Build history of the part. All positions in model axes, mm. Face numbers are marked on the shaded views. A direction names the side the tool comes from. Give positions to 0.01 mm unless a question says otherwise; leave off trailing zeros. Order: outer loops, then holes, each group sorted by start corner. A loop starts at its lowest first (then second) coordinate and runs counter-clockwise, first axis right, second up. Notation, with made-up numbers: (58, -33.5) - (109, -33.5) arc R18 ccw to (109, -16.5) - close; hole circle Ø3 at (16.5, 53). An arc over 180 degrees is marked (long way). Answer in a Markdown table with one row per item.
```python
from build123d import *

# Parameters (mm, degrees)
F0_R     = 25
F1_DEPTH = 1.9
F2_R     = 1.05
F3_DEPTH = 25.4
F5_DEPTH = 5


with BuildPart() as f1:
    # F0 (on Top) → F1 (new body)
    with BuildSketch(Plane.XY):
        Circle(F0_R)
    extrude(amount=F1_DEPTH)

    # F2 (on Top) → F3 (cut)
    with BuildSketch(Plane.XY):
        Circle(F2_R)
    extrude(amount=F3_DEPTH, mode=Mode.SUBTRACT)

    # F4 (on face) → F5 (join)
    with BuildSketch(Plane.XY.offset(1.9)):
        with BuildLine():
            ThreePointArc((-8.4449654791, 14.1750681853), (-7.8625386646, 14.5062223114), (-7.267148147, 14.8134586714))
            Line((-7.267148147, 14.8134586714), (-6.6282985683, 17.5245980034))
            Line((-6.6282985683, 17.5245980034), (-13.8357791201, 20.8223729709))
            ThreePointArc((-13.8357791201, 20.8223729709), (-14.3152843529, 20.4956735409), (-14.7870786227, 20.1579340659))
            Line((-14.7870786227, 20.1579340659), (-7.7896110966, 16.9562503322))
            Line((-7.7896110966, 16.9562503322), (-8.4449654791, 14.1750681853))
        make_face()
        with BuildLine():
            ThreePointArc((-1.4583194007, 16.4354283341), (-0.7898885826, 16.4810823682), (-0.1201554013, 16.4995624996))
            Line((-0.1201554013, 16.4995624996), (1.631747451, 18.6650281904))
            Line((1.631747451, 18.6650281904), (-3.4311172084, 24.7634293809))
            ThreePointArc((-3.4311172084, 24.7634293809), (-4.0048860655, 24.6771328886), (-4.5764976809, 24.5775439981))
            Line((-4.5764976809, 24.5775439981), (0.3388442045, 18.6568392545))
            Line((0.3388442045, 18.6568392545), (-1.4583194007, 16.4354283341))
        make_face()
        with BuildLine():
            ThreePointArc((5.8171647201, 15.4405503341), (6.4392086206, 15.1916619348), (7.0506355953, 14.917725621))
            Line((7.0506355953, 14.917725621), (9.5686058756, 16.1086206327))
            Line((9.5686058756, 16.1086206327), (7.6531195462, 23.7997848984))
            ThreePointArc((7.6531195462, 23.7997848984), (7.0987290239, 23.9709834226), (6.5405147537, 24.1292699176))
            Line((6.5405147537, 24.1292699176), (8.4001872552, 16.6622123514))
            Line((8.4001872552, 16.6622123514), (5.8171647201, 15.4405503341))
        make_face()
        with BuildLine():
            ThreePointArc((11.9404880253, 11.3874819745), (12.3929415847, 10.8933465417), (12.8249617418, 10.3812502291))
            Line((12.8249617418, 10.3812502291), (15.6102845553, 10.3617031995))
            Line((15.6102845553, 10.3617031995), (17.2215621154, 18.1223011316))
            ThreePointArc((17.2215621154, 18.1223011316), (16.7963537699, 18.5170867049), (16.3620980272, 18.9018980039))
            Line((16.3620980272, 18.9018980039), (14.7977701984, 11.3674299434))
            Line((14.7977701984, 11.3674299434), (11.9404880253, 11.3874819745))
        make_face()
        with BuildLine():
            ThreePointArc((15.6988512365, 5.0789831515), (15.8921004786, 4.4374702679), (16.0591469276, 3.7886409118))
            Line((16.0591469276, 3.7886409118), (18.5601549312, 2.5625233696))
            Line((18.5601549312, 2.5625233696), (23.379063099, 8.8554733703))
            ThreePointArc((23.379063099, 8.8554733703), (23.167254658, 9.3956538681), (22.9429671184, 9.9307733739))
            Line((22.9429671184, 9.9307733739), (18.2644732712, 3.8211886228))
            Line((18.2644732712, 3.8211886228), (15.6988512365, 5.0789831515))
        make_face()
        with BuildLine():
            Line((18.1136734135, -4.4818859684), (16.3478644266, -2.2354705742))
            ThreePointArc((16.3478644266, -2.2354705742), (16.2436339688, -2.8973014145), (16.1126211118, -3.5543552028))
            Line((16.1126211118, -3.5543552028), (17.8339589977, -5.7441956409))
            Line((17.8339589977, -5.7441956409), (24.9060539105, -2.1652894973))
            ThreePointArc((24.9060539105, -2.1652894973), (24.9495966334, -1.5867034474), (24.9797001948, -1.0072627157))
            Line((24.9797001948, -1.0072627157), (18.1136734135, -4.4818859684))
        make_face()
        with BuildLine():
            Line((14.3752383867, -11.8972680768), (13.7589825736, -9.1071619365))
            ThreePointArc((13.7589825736, -9.1071619365), (13.3779165365, -9.6582270186), (12.9747930765, -10.1933676782))
            Line((12.9747930765, -10.1933676782), (13.5755287655, -12.9132062568))
            Line((13.5755287655, -12.9132062568), (21.5000952923, -12.7571902244))
            ThreePointArc((21.5000952923, -12.7571902244), (21.7903650088, -12.2547946855), (22.0688972917, -11.7457980712))
            Line((22.0688972917, -11.7457980712), (14.3752383867, -11.8972680768))
        make_face()
        with BuildLine():
            Line((7.7896110966, -16.9562503322), (8.4449654791, -14.1750681853))
            ThreePointArc((8.4449654791, -14.1750681853), (7.8625386646, -14.5062223114), (7.267148147, -14.8134586714))
            Line((7.267148147, -14.8134586714), (6.6282985683, -17.5245980034))
            Line((6.6282985683, -17.5245980034), (13.8357791201, -20.8223729709))
            ThreePointArc((13.8357791201, -20.8223729709), (14.3152843529, -20.4956735409), (14.7870786227, -20.1579340659))
            Line((14.7870786227, -20.1579340659), (7.7896110966, -16.9562503322))
        make_face()
        with BuildLine():
            Line((-0.3388442045, -18.6568392545), (1.4583194007, -16.4354283341))
            ThreePointArc((1.4583194007, -16.4354283341), (0.7898885826, -16.4810823682), (0.1201554013, -16.4995624996))
            Line((0.1201554013, -16.4995624996), (-1.631747451, -18.6650281904))
            Line((-1.631747451, -18.6650281904), (3.4311172084, -24.7634293809))
            ThreePointArc((3.4311172084, -24.7634293809), (4.0048860655, -24.6771328886), (4.5764976809, -24.5775439981))
            Line((4.5764976809, -24.5775439981), (-0.3388442045, -18.6568392545))
        make_face()
        with BuildLine():
            Line((-8.4001872552, -16.6622123514), (-5.8171647201, -15.4405503341))
            ThreePointArc((-5.8171647201, -15.4405503341), (-6.4392086206, -15.1916619348), (-7.0506355953, -14.917725621))
            Line((-7.0506355953, -14.917725621), (-9.5686058756, -16.1086206327))
            Line((-9.5686058756, -16.1086206327), (-7.6531195462, -23.7997848984))
            ThreePointArc((-7.6531195462, -23.7997848984), (-7.0987290239, -23.9709834226), (-6.5405147537, -24.1292699176))
            Line((-6.5405147537, -24.1292699176), (-8.4001872552, -16.6622123514))
        make_face()
        with BuildLine():
            Line((-14.7977701984, -11.3674299434), (-11.9404880253, -11.3874819745))
            ThreePointArc((-11.9404880253, -11.3874819745), (-12.3929415847, -10.8933465417), (-12.8249617418, -10.3812502291))
            Line((-12.8249617418, -10.3812502291), (-15.6102845553, -10.3617031995))
            Line((-15.6102845553, -10.3617031995), (-17.2215621154, -18.1223011316))
            ThreePointArc((-17.2215621154, -18.1223011316), (-16.7963537699, -18.5170867049), (-16.3620980272, -18.9018980039))
            Line((-16.3620980272, -18.9018980039), (-14.7977701984, -11.3674299434))
        make_face()
        with BuildLine():
            Line((-18.2644732712, -3.8211886228), (-15.6988512365, -5.0789831515))
            ThreePointArc((-15.6988512365, -5.0789831515), (-15.8921004786, -4.4374702679), (-16.0591469276, -3.7886409118))
            Line((-16.0591469276, -3.7886409118), (-18.5601549312, -2.5625233696))
            Line((-18.5601549312, -2.5625233696), (-23.379063099, -8.8554733703))
            ThreePointArc((-23.379063099, -8.8554733703), (-23.167254658, -9.3956538681), (-22.9429671184, -9.9307733739))
            Line((-22.9429671184, -9.9307733739), (-18.2644732712, -3.8211886228))
        make_face()
        with BuildLine():
            ThreePointArc((-16.3478644266, 2.2354705742), (-16.2436339688, 2.8973014145), (-16.1126211118, 3.5543552028))
            Line((-16.1126211118, 3.5543552028), (-17.8339589977, 5.7441956409))
            Line((-17.8339589977, 5.7441956409), (-24.9060539105, 2.1652894973))
            ThreePointArc((-24.9060539105, 2.1652894973), (-24.9495966334, 1.5867034474), (-24.9797001948, 1.0072627157))
            Line((-24.9797001948, 1.0072627157), (-18.1136734135, 4.4818859684))
            Line((-18.1136734135, 4.4818859684), (-16.3478644266, 2.2354705742))
        make_face()
        with BuildLine():
            ThreePointArc((-13.7589825736, 9.1071619365), (-13.3779165365, 9.6582270186), (-12.9747930765, 10.1933676782))
            Line((-12.9747930765, 10.1933676782), (-13.5755287655, 12.9132062568))
            Line((-13.5755287655, 12.9132062568), (-21.5000952923, 12.7571902244))
            ThreePointArc((-21.5000952923, 12.7571902244), (-21.7903650088, 12.2547946855), (-22.0688972917, 11.7457980712))
            Line((-22.0688972917, 11.7457980712), (-14.3752383867, 11.8972680768))
            Line((-14.3752383867, 11.8972680768), (-13.7589825736, 9.1071619365))
        make_face()
    extrude(amount=F5_DEPTH)


solid = f1.part
```
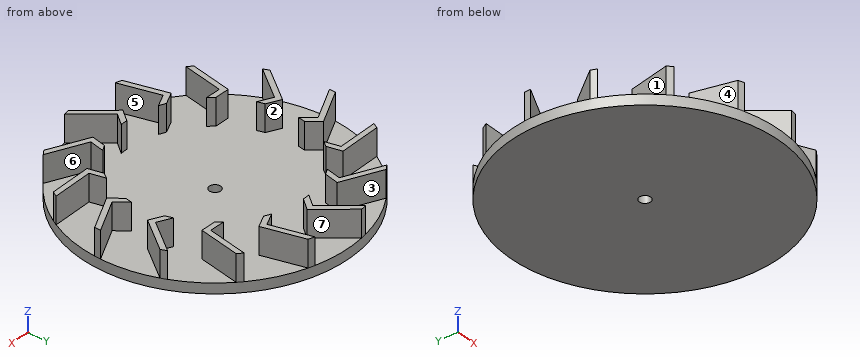
1. Cut at C-C on x = -4. Write the cut outline in (y, z).
Check result:
| item | result |
|---|---|
| outline | (-24.68, 0) - (24.68, 0) - (24.68, 6.9) - (23.88, 6.9) - (23.88, 1.9) - (-24.68, 1.9) - close |
2. Drop flat-ended pins along their axis: P1, Ø2, axis at y = -5.5, z = 6, coming from the -X side; P2, Ø2, axis at x = -15.5, z = 3.5, coming from the -Y side; P3, Ø2, axis at x = -18, z = 2.5, coming from the +Y side. Give the stop position or say it passes through.
Check result:
| item | result |
|---|---|
| P1 | stops at x = -21.58 |
| P2 | stops at y = -18.9 |
| P3 | stops at y = 18.14 |
3. Probe line 1 (Y direction, x = 0, z = 1.5); line 2 (X direction, y = 4, z = 4.5). List the from-to ranges inside material, lowest first.
Check result:
| item | result |
|---|---|
| line 1 | y = -25 to -1.05, 1.05 to 25 |
| line 2 | x = -21.28 to -19.07, -17.73 to -16.46, 16.01 to 17.9, 18.4 to 19.66 |
4. Which spindle directions (+Z, -Z, +X, -X, +Y, -Y) get a long thin tool onto all of the face, cutting with end or side? Do the marked faces 1, 2 and 3. Say none if no direction does.
Check result:
| item | result |
|---|---|
| face 1 | +Z, -X |
| face 2 | +Z |
| face 3 | +Z, +Y |
5. Two-plate mould, pull along Y, no slides. Class the marked faces 4, 5, 6 and 7: +Y half, -Y half, draft (parallel to the pull), parting line (faces both ways), or undercut.
Check result:
| item | result |
|---|---|
| face 4 | -Y half |
| face 5 | undercut |
| face 6 | undercut |
| face 7 | +Y half |
6. Cut at B-B on z = 5.5. Count the separate pieces of the cut face and the enclosed holes in it, and give its area (3 significant figures).
Check result:
| item | result |
|---|---|
| separate pieces | 14 |
| enclosed holes | 0 |
| area | 149 mm² |
7. Cut at D-D on x = -10.5. Write the cut outline in (y, z), and give its area (3 significant figures).
Check result:
| item | result |
|---|---|
| outline | (-22.69, 0) - (22.69, 0) - (22.69, 1.9) - (19.3, 1.9) - (19.3, 6.9) - (18.2, 6.9) - (18.2, 1.9) - (-22.69, 1.9) - close |
| area | 91.7 mm² |
8. Cut at A-A on y = 0. Write the cut outline in (x, z).
Check result:
| item | result |
|---|---|
| outline | (-25, 0) - (-1.05, 0) - (-1.05, 1.9) - (-25, 1.9) - close; (1.05, 0) - (25, 0) - (25, 1.9) - (1.05, 1.9) - close |
